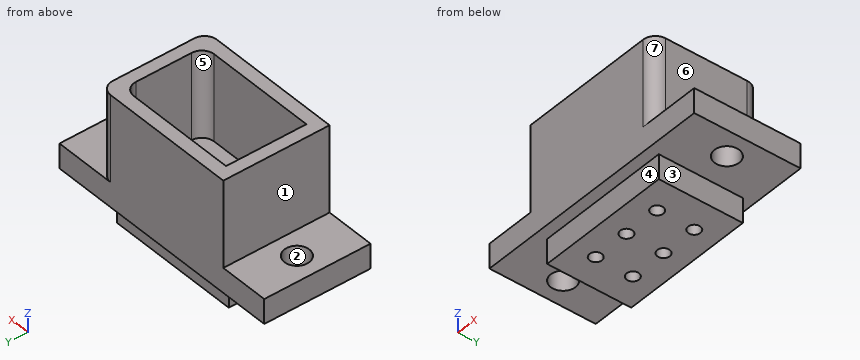
```python
from build123d import *

# Parameters (mm, degrees)
SKETCH_1_W      = 10.9
SKETCH_1_H      = 6.8
SKETCH_1_R      = 0.5
EXTRUDE_1_DEPTH = 2
SKETCH_2_W      = 20
SKETCH_2_H      = 8.6
SKETCH_2_R      = 1
SKETCH_2_R_2    = 0.5
EXTRUDE_2_DEPTH = 2
EXTRUDE_3_DEPTH = 7


with BuildPart() as part:
    # 草图1 → 凸台-拉伸1 (new body)
    with BuildSketch(Plane.XY):
        Rectangle(SKETCH_1_W, SKETCH_1_H)
        with Locations((-3, 1.5)):
            Circle(SKETCH_1_R, mode=Mode.SUBTRACT)
        with Locations((0, 1.5)):
            Circle(SKETCH_1_R, mode=Mode.SUBTRACT)
        with Locations((3, 1.5)):
            Circle(SKETCH_1_R, mode=Mode.SUBTRACT)
        with Locations((0, -1.5)):
            Circle(SKETCH_1_R, mode=Mode.SUBTRACT)
        with Locations((3, -1.5)):
            Circle(SKETCH_1_R, mode=Mode.SUBTRACT)
        with Locations((-3, -1.5)):
            Circle(SKETCH_1_R, mode=Mode.SUBTRACT)
    extrude(amount=EXTRUDE_1_DEPTH)

    # 草图2 → 凸台-拉伸2 (add)
    with BuildSketch(Plane.XY.offset(2)):
        Rectangle(SKETCH_2_W, SKETCH_2_H)
        with Locations((-8, 0)):
            Circle(SKETCH_2_R, mode=Mode.SUBTRACT)
        with Locations(Location((8, 0, 0), (0, 0, 180))):
            Circle(SKETCH_2_R, mode=Mode.SUBTRACT)
        with Locations((3, 1.5)):
            Circle(SKETCH_2_R_2, mode=Mode.SUBTRACT)
        with Locations((3, -1.5)):
            Circle(SKETCH_2_R_2, mode=Mode.SUBTRACT)
        with Locations((0, -1.5)):
            Circle(SKETCH_2_R_2, mode=Mode.SUBTRACT)
        with Locations((0, 1.5)):
            Circle(SKETCH_2_R_2, mode=Mode.SUBTRACT)
        with Locations((-3, -1.5)):
            Circle(SKETCH_2_R_2, mode=Mode.SUBTRACT)
        with Locations((-3, 1.5)):
            Circle(SKETCH_2_R_2, mode=Mode.SUBTRACT)
    extrude(amount=EXTRUDE_2_DEPTH)

    # 草图3 → 凸台-拉伸3 (add)
    with BuildSketch(Plane.XY.offset(4)):
        with BuildLine():
            Line((5, 4.3), (-6, 4.3))
            Line((-6, 4.3), (-6, -4.3))
            Line((-6, -4.3), (5, -4.3))
            ThreePointArc((5, -4.3), (5.707106781, -4.007106781), (6, -3.3))
            Line((6, -3.3), (6, 3.3))
            ThreePointArc((6, 3.3), (5.707106781, 4.007106781), (5, 4.3))
        make_face()
        with BuildLine():
            Line((-5, -3.25), (-5, 3.25))
            Line((-5, 3.25), (4, 3.25))
            ThreePointArc((4, 3.25), (4.707106781, 2.957106781), (5, 2.25))
            Line((5, 2.25), (5, -2.25))
            ThreePointArc((5, -2.25), (4.707106781, -2.957106781), (4, -3.25))
            Line((4, -3.25), (-5, -3.25))
        make_face(mode=Mode.SUBTRACT)
    extrude(amount=EXTRUDE_3_DEPTH)


solid = part.part
```
Design review of the part built by this model. Coordinates are the model's own, in mm. Face numbers are marked on the shaded views. A direction names the side the tool comes from. Give positions to 0.01 mm unless a question says otherwise; leave off trailing zeros. Write each loop counter-clockwise with the first axis right and the second up, starting at its lowest first coordinate (ties: lowest second). Pieces come first, ordered by that corner, then holes.
(1) Add section D-D (z = 6.75). Give the boundary of the cut face in (x, y), and give its area (3 significant figures).
Checked values:
outline: (-6, -4.3) - (5, -4.3) arc R1 ccw to (6, -3.3) - (6, 3.3) arc R1 ccw to (5, 4.3) - (-6, 4.3) - close; hole (-5, -3.25) - (4, -3.25) arc R1 ccw to (5, -2.25) - (5, 2.25) arc R1 ccw to (4, 3.25) - (-5, 3.25) - close
area: 38.2 mm2
(2) Tool access review of the marked faces 4, 5, 6 and 7: name each direction out of +Z, -Z, +X, -X, +Y, -Y from which nothing blocks a thin tool from reaching the whole face with its end or side.
Checked values:
face 4: -Z, +X, -X, -Y
face 5: +Z
face 6: +Z, +X, +Y, -Y
face 7: +Z, +X, -Y
(3) Wall thickness on line 1 along Y through (x, z) = (0, 1.75); line 2 along Y through (x, z) = (3, 2.75); line 3 along X through (y, z) = (1.25, 5.5): over which ranges is each line inside the solid? List them lowest first.
Checked values:
line 1: y = -3.4 to -2, -1 to 1, 2 to 3.4
line 2: y = -4.3 to -2, -1 to 1, 2 to 4.3
line 3: x = -6 to -5, 5 to 6
(4) Mouldability with a two-part tool opening along X and no side actions: class the marked faces 1, 2 and 3 as +X half, -X half, draft (parallel to the pull), parting line (faces both ways), or undercut.
Checked values:
face 1: -X half
face 2: undercut
face 3: +X half
(5) Add section A-A (x = 8). Give the boundary of the cut face in (y, z), and give its area (3 significant figures).
Checked values:
outline: (-4.3, 2) - (-1, 2) - (-1, 4) - (-4.3, 4) - close; (1, 2) - (4.3, 2) - (4.3, 4) - (1, 4) - close
area: 13.2 mm2
(6) Add section B-B (y = 1.5). Give the boundary of the cut face in (x, z), and give its area (3 significant figures).
Checked values:
outline: (-10, 2) - (-5.45, 2) - (-5.45, 0) - (-3.5, 0) - (-3.5, 4) - (-5, 4) - (-5, 11) - (-6, 11) - (-6, 4) - (-10, 4) - close; (-2.5, 0) - (-0.5, 0) - (-0.5, 4) - (-2.5, 4) - close; (0.5, 0) - (2.5, 0) - (2.5, 4) - (0.5, 4) - close; (3.5, 0) - (5.45, 0) - (5.45, 2) - (10, 2) - (10, 4) - (6, 4) - (6, 11) - (5, 11) - (5, 4) - (3.5, 4) - close
area: 63.8 mm2
(7) Clearance check with flat-ended pins moving along their axes: pin 1 Ø3 at (x, y) = (8, 0) entering from -Z; pin 2 Ø1 at (x, z) = (2, 1) entering from +Y; pin 3 Ø2 at (x, y) = (-7.5, -0.5) entering from +Z. State where each tip first meets the part, or that it passes through.
Checked values:
pin 1: stops at z = 2
pin 2: stops at y = 3.4
pin 3: stops at z = 4
(8) Add section C-C (x = 0). Give the boundary of the cut face in (y, z), and give its area (3 significant figures).
Checked values:
outline: (-4.3, 2) - (-3.4, 2) - (-3.4, 0) - (-2, 0) - (-2, 4) - (-3.25, 4) - (-3.25, 11) - (-4.3, 11) - close; (-1, 0) - (1, 0) - (1, 4) - (-1, 4) - close; (2, 0) - (3.4, 0) - (3.4, 2) - (4.3, 2) - (4.3, 11) - (3.25, 11) - (3.25, 4) - (2, 4) - close
area: 37.5 mm2
